Read the model definition and answer for the solid it produces. Units are mm, in the model's axes. Face numbers are marked on the shaded views. A direction names the side the tool comes from. Coordinates: 2 decimals unless noted, no trailing zeros. Write each loop counter-clockwise with the first axis right and the second up, starting at its lowest first coordinate (ties: lowest second). Pieces come first, ordered by that corner, then holes. Notation, with made-up numbers: (65, -34) - (100, -34) arc R17 ccw to (100, -25) - close; hole circle Ø3 at (-29.75, 35). An arc over 180 degrees is marked (long way). Return JSON: item names as keys, results as strings.
```python
from build123d import *

# Parameters (mm, degrees)
SKETCH2_R             = 21
SKETCH2_R_2           = 16
BOSS_EXTRUDE3_DEPTH   = 10
SKETCH2_R_3           = 12.5
SKETCH2_R_4           = 6.25
BOSS_EXTRUDE3_2_DEPTH = 10
BOSS_EXTRUDE4_DEPTH   = 6
CUT_EXTRUDE2_START    = -6
CUT_EXTRUDE2_DEPTH    = 132.802456026
CUT_EXTRUDE3_START    = 6
CUT_EXTRUDE3_DEPTH    = 132.802456026


with BuildPart() as part:
    # Sketch2 → Boss-Extrude3 (new, symmetric)
    with BuildSketch(Plane.XY):
        Circle(SKETCH2_R)
        Circle(SKETCH2_R_2, mode=Mode.SUBTRACT)
    extrude(amount=BOSS_EXTRUDE3_DEPTH, both=True)



with BuildPart() as body_2:
    # Sketch2 → Boss-Extrude3 2 (new, symmetric)
    with BuildSketch(Plane.XY):
        with Locations((0, 120)):
            Circle(SKETCH2_R_3)
        with Locations((0, 120)):
            Circle(SKETCH2_R_4, mode=Mode.SUBTRACT)
    extrude(amount=BOSS_EXTRUDE3_2_DEPTH, both=True)


with BuildPart() as part_1:
    add(part.part)

    add(body_2.part)  # Boss-Extrude4 merges body 2
    # Sketch2_6 → Boss-Extrude4 (add, symmetric)
    with BuildSketch(Plane.XY):
        with BuildLine():
            ThreePointArc((0, 107.5), (-2.46047965, 107.744550604), (-4.824685415, 108.468633617))
            Line((-4.824685415, 108.468633617), (-9.743614629, 73.468633617))
            ThreePointArc((-9.743614629, 73.468633617), (-14.942721631, 38.479711201), (-20.693090304, 3.577151615))
            ThreePointArc((-20.693090304, 3.577151615), (-13.525528013, 16.064248876), (0, 21))
            Line((0, 21), (0, 107.5))
        make_face()
        with BuildLine():
            ThreePointArc((4.824685415, 108.468633617), (2.46047965, 107.744550604), (0, 107.5))
            Line((0, 107.5), (0, 21))
            ThreePointArc((0, 21), (13.525528013, 16.064248876), (20.693090304, 3.577151615))
            ThreePointArc((20.693090304, 3.577151615), (14.942721631, 38.479711201), (9.743614629, 73.468633617))
            Line((9.743614629, 73.468633617), (4.824685415, 108.468633617))
        make_face()
        with BuildLine():
            ThreePointArc((17, -12.328828006), (9.541871197, -18.707022587), (0, -21))
            Line((0, -21), (0, -24.328828006))
            Line((0, -24.328828006), (17, -24.328828006))
            Line((17, -24.328828006), (17, -12.328828006))
        make_face()
        with BuildLine():
            ThreePointArc((0, -21), (-9.541871197, -18.707022587), (-17, -12.328828006))
            Line((-17, -12.328828006), (-17, -24.328828006))
            Line((-17, -24.328828006), (0, -24.328828006))
            Line((0, -24.328828006), (0, -21))
        make_face()
        with BuildLine():
            Line((6.25, 135.825317547), (0, 135.825317547))
            Line((0, 135.825317547), (0, 132.5))
            ThreePointArc((0, 132.5), (3.235238064, 132.074072829), (6.25, 130.825317547))
            Line((6.25, 130.825317547), (6.25, 135.825317547))
        make_face()
        with BuildLine():
            Line((0, 132.5), (0, 135.825317547))
            Line((0, 135.825317547), (-6.25, 135.825317547))
            Line((-6.25, 135.825317547), (-6.25, 130.825317547))
            ThreePointArc((-6.25, 130.825317547), (-3.235238064, 132.074072829), (0, 132.5))
        make_face()
    extrude(amount=BOSS_EXTRUDE4_DEPTH, both=True)

    # Sketch3 → Cut-Extrude2 (cut, through all)
    with BuildSketch(Plane(origin=(0, 0, 0), x_dir=(0, 0, -1), z_dir=(1, 0, 0)).offset(CUT_EXTRUDE2_START)):
        with BuildLine():
            Line((4, 100), (4, 38))
            ThreePointArc((4, 38), (0, 34), (-4, 38))
            Line((-4, 38), (-4, 100))
            ThreePointArc((-4, 100), (0, 104), (4, 100))
        make_face()
    extrude(amount=-CUT_EXTRUDE2_DEPTH, mode=Mode.SUBTRACT)

    # Sketch3_2 → Cut-Extrude3 (cut, through all)
    with BuildSketch(Plane(origin=(0, 0, 0), x_dir=(0, 0, -1), z_dir=(1, 0, 0)).offset(CUT_EXTRUDE3_START)):
        with BuildLine():
            Line((4, 100), (4, 38))
            ThreePointArc((4, 38), (0, 34), (-4, 38))
            Line((-4, 38), (-4, 100))
            ThreePointArc((-4, 100), (0, 104), (4, 100))
        make_face()
    extrude(amount=CUT_EXTRUDE3_DEPTH, mode=Mode.SUBTRACT)


solid = part_1.part
```
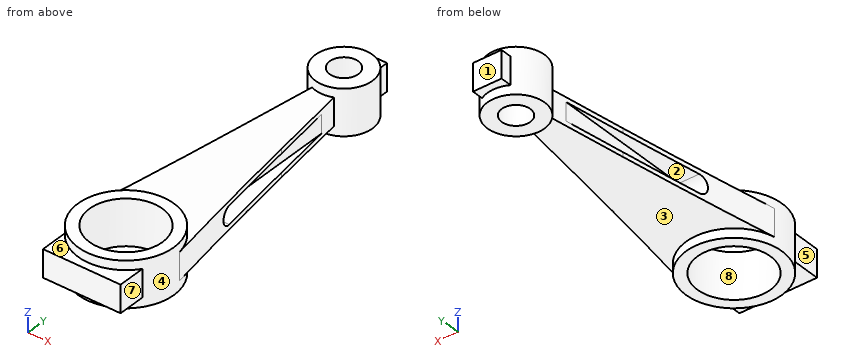
(1) Straight lines are drawn through the part: line 1 (Y direction, x = 0, z = 0.5); line 2 (Z direction, x = 7.5, y = 56); line 3 (Y direction, x = 9.5, z = -6.5). For each, find the intervals that lie inside material, in ascending order. Write a range as from..to.
Answer:
{"line 1": "-24.33..-16, 16..113.75, 126.25..135.83", "line 2": "-6..-4, 4..6", "line 3": "-18.73..-12.87, 12.87..18.73, 111.88..128.12"}
(2) Determine the mould class of the marked faces 1, 2 and 3 for opening direction Z: +Z half, -Z half, draft (parallel to the pull), parting line (faces both ways), or undercut.
Answer:
{"face 1": "draft", "face 2": "undercut", "face 3": "-Z half"}
(3) A cutting plane is placed at C-C (x = 2). Determine the outline of the cut face in (y, z).
Answer:
{"outline": "(-24.33, -6) - (-20.9, -6) - (-20.9, -10) - (-15.87, -10) - (-15.87, 10) - (-20.9, 10) - (-20.9, 6) - (-24.33, 6) - close; (15.87, -10) - (20.9, -10) - (20.9, -6) - (107.66, -6) - (107.66, -10) - (114.08, -10) - (114.08, 10) - (107.66, 10) - (107.66, 6) - (20.9, 6) - (20.9, 10) - (15.87, 10) - close; (125.92, -10) - (132.34, -10) - (132.34, -6) - (135.83, -6) - (135.83, 6) - (132.34, 6) - (132.34, 10) - (125.92, 10) - close"}
(4) A cutting plane is placed at B-B (z = 0). Determine the outline of the cut face in (x, y).
Answer:
{"outline": "(-20.69, 3.58) arc R21 ccw to (-17, -12.33) - (-17, -24.33) - (17, -24.33) - (17, -12.33) arc R21 ccw to (20.69, 3.58) arc R2242.45 cw to (15.65, 34) - (6, 34) - (6, 100.11) - (4.82, 108.47) arc R12.5 ccw to (6.25, 130.83) - (6.25, 135.83) - (-6.25, 135.83) - (-6.25, 130.83) arc R12.5 ccw to (-4.82, 108.47) - (-6, 100.11) - (-6, 34) - (-15.65, 34) arc R2242.45 cw to start; hole circle Ø32 at (0, 0); hole circle Ø12.5 at (0, 120)"}
(5) A cutting plane is placed at A-A (y = 0). Determine the outline of the cut face in (x, z).
Answer:
{"outline": "(-21, -10) - (-16, -10) - (-16, 10) - (-21, 10) - close; (16, -10) - (21, -10) - (21, 10) - (16, 10) - close"}
(6) Which of the six approach directions +Z, -Z, +X, -X, +Y, -Y give full straight-line access (tool end or side, diameter ignored) to the marked faces 4, 5, 6, 7 and 8?
Answer:
{"face 4": "none", "face 5": "+Z, -Z, -X, -Y", "face 6": "+Z, -Y", "face 7": "+Z, -Z, +X, -Y", "face 8": "+Z, -Z"}
(7) A cutting plane is placed at D-D (y = 120). Determine the outline of the cut face in (x, z), and give its area (3 significant figures).
Answer:
{"outline": "(-12.5, -10) - (-6.25, -10) - (-6.25, 10) - (-12.5, 10) - close; (6.25, -10) - (12.5, -10) - (12.5, 10) - (6.25, 10) - close", "area": "250 mm²"}
(8) Flat-ended cylindrical pins translate along their axes: P1, Ø10, axis at x = -11.5, y = 66.5, coming from the -Z side; P2, Ø10, axis at x = -8.5, y = 63, coming from the +Z side; P3, Ø4, axis at y = 17, z = 5.5, coming from the -X side. Find the tip coordinate at first contact, or state that the pin passes through.
Answer:
{"P1": "z = -6", "P2": "z = 6", "P3": "x = -18.75"}
